Part model, mm, in its own coordinate system. Face numbers are marked on the shaded views. Round coordinates to 2 decimals unless told otherwise and drop trailing zeros. Loops run counter-clockwise (first coordinate to the right, second up) from the corner with the lowest first, then second, coordinate; pieces in that order, holes last. Notation, with made-up numbers: (-25, 74.25) -> (30, 74.25) arc R18 ccw to (30, 85.25) -> close; hole circle Ø8 at (43, -8). An arc over 180 degrees is marked (long way). Use a Markdown table: item, result. Add a question column.
Item 1: Flat gauge pins, fed straight in: pin 1 (2 mm diameter, centred on x = 2, z = 0, fed in from +Y) (3 decimals); pin 2 (5 mm diameter, centred on x = 8, y = 4.5, fed in from -Z). Where does each tip first touch, or does it go through?
Item 2: Cut at C-C, the plane z = 5. List the corners of the cut face in (x, y).
Item 3: Probe line 1 (X direction, y = 0.5, z = 2.5); line 2 (Y direction, x = 8, z = -5.5); line 3 (X direction, y = -3.5, z = -1). List the from-to ranges inside material, lowest first. Write a range as [from, to].
Item 4: Cut at B-B, the plane y = -3.75. List the corners of the cut face in (x, z), plus the area to 3 significant figures.
Item 5: Two-plate mould, pull along Y, no slides. Class the marked faces 1 and 2: pulls with the +Y half, pulls with the -Y half, needs draft (parallel to the pull), parting line crosses it, or undercut.
Item 6: Cut at D-D, the plane y = 2.75. State how many separate pieces and enclosed holes the cut face has, plus the area to 3 significant figures.
Item 7: Cut at A-A, the plane x = 5.75. List the corners of the cut face in (y, z), plus the area to 3 significant figures.
```python
from build123d import *

# Parameters (mm, degrees)
THREAD1_PITCH = 1.27


with BuildPart() as part:
    # Sketch1 → Revolve1 (revolve)
    with BuildSketch(Plane.XY, mode=Mode.PRIVATE) as revolve1_sk:
        Polygon((0, 0), (0, 3.175), (3.81, 3.175), (3.81, 6.35), (10.16, 6.35), (10.16, 0), align=None)
    revolve(revolve1_sk.sketch.rotate(Axis((10.16, 0, 0), (-1, 0, 0)), 90), axis=Axis((10.16, 0, 0), (-1, 0, 0)))

    # Thread1: the profile of Thread Profile1 profile screwed along a right-hand helix of 3 turns, 8 arcs to a turn; built about Z, then put on its axis
    thread1_z = Axis((0, 0, 0), (0, 0, 1))
    thread1_corners = [(3.1753, 0, -0.000173205), (3.1753, 0, 1.111423202), (2.487592339, 0, 0.714374998), (2.487592339, 0, 0.396874998)]
    with BuildLine(mode=Mode.PRIVATE) as thread1_profile:
        Line(thread1_corners[0], thread1_corners[1])
        Line(thread1_corners[1], thread1_corners[2])
        Line(thread1_corners[2], thread1_corners[3])
        Line(thread1_corners[3], thread1_corners[0])
    thread1_cap = Face(thread1_profile.wire())
    thread1_turn_angles = [0, 22.5, 45, 67.5, 90, 112.5, 135, 157.5, 180, 202.5, 225, 247.5, 270, 292.5, 315, 337.5, 360]
    thread1_turn_weights = [1, 0.9238795325112867, 1, 0.9238795325112867, 1, 0.9238795325112867, 1, 0.9238795325112867, 1, 0.9238795325112867, 1, 0.9238795325112867, 1, 0.9238795325112867, 1, 0.9238795325112867, 1]
    thread1_turn_rails = [Edge.make_bspline([Vector(p[0], p[1], 0).rotate(thread1_z, thread1_turn_angles[k]) / thread1_turn_weights[k] + Vector(0, 0, p[2] + THREAD1_PITCH * thread1_turn_angles[k] / 360) for k in range(17)], [0, 0, 0, 1, 1, 2, 2, 3, 3, 4, 4, 5, 5, 6, 6, 7, 7, 8, 8, 8], 2, thread1_turn_weights) for p in thread1_corners]
    thread1_turn_sides = [Face.make_surface_from_curves(thread1_turn_rails[p[0]], thread1_turn_rails[p[1]]) for p in [(0, 1), (1, 2), (2, 3), (3, 0)]]
    thread1 = Plane(origin=(3.81, 0, 0), x_dir=(0, 0, 1), z_dir=(-1, 0, 0)) * Solid(Shell([*[p.moved(Location((0, 0, THREAD1_PITCH * i))) for i in range(3) for p in thread1_turn_sides], thread1_cap, thread1_cap.rotate(thread1_z, 1080).moved(Location((0, 0, THREAD1_PITCH * 1080 / 360)))]))
    add(thread1, mode=Mode.SUBTRACT)


solid = part.part
```
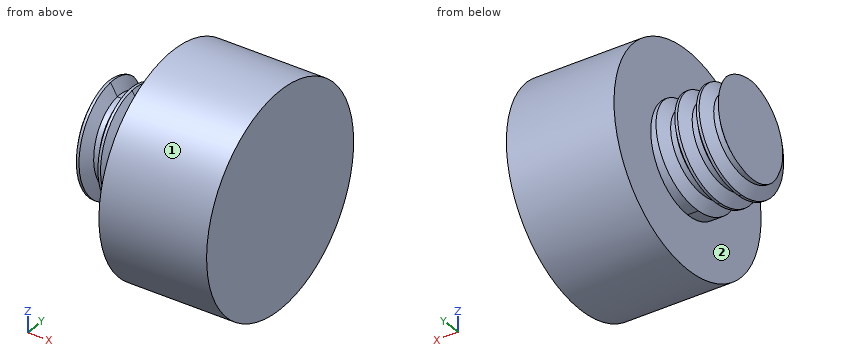
A:
| question | item | result |
|---|---|---|
| 1 | pin 1 | stops at y = 3.175 |
| 1 | pin 2 | stops at z = -6.03 |
| 2 | outline | (3.81, -3.91) -> (10.16, -3.91) -> (10.16, 3.91) -> (3.81, 3.91) -> close |
| 3 | line 1 | x = [0, 0.48], [0.87, 1.75], [2.14, 3.02], [3.41, 10.16] |
| 3 | line 2 | y = [-3.17, 3.17] |
| 3 | line 3 | x = [3.81, 10.16] |
| 4 | outline | (3.81, -5.12) -> (10.16, -5.12) -> (10.16, 5.12) -> (3.81, 5.12) -> close |
| 4 | area | 65.1 mm^2 |
| 5 | face 1 | parting line crosses it |
| 5 | face 2 | needs draft |
| 6 | separate pieces | 4 |
| 6 | enclosed holes | 0 |
| 6 | area | 77.4 mm^2 |
| 7 | outline | circle Ø12.7 at (0, 0) |
| 7 | area | 127 mm^2 |
